```python
from build123d import *

# Parameters (mm, degrees)
RESSALTO_EXTRUS_O1_DEPTH = 102
ESBO_O3_R                = 1.5
CORTE_EXTRUS_O2_DEPTH    = 10


with BuildPart() as part:
    # Esboço1 → Ressalto-extrusão1 (new body)
    with BuildSketch(Plane.XY):
        Polygon((-21.132279289, 13.382352941), (-21.132279289, -6.617647059), (78.834377283, -9.19981162), align=None)
    extrude(amount=RESSALTO_EXTRUS_O1_DEPTH)

    # Esboço3 → Corte-extrusão2 (cut)
    with BuildSketch(Plane(origin=(-0.184911664, -7.158722975, 0), x_dir=(0.999666566, -0.025821646, 0), z_dir=(-0.025821646, -0.999666566, 0))):
        with Locations((4.045645474, 25)):
            Circle(ESBO_O3_R)
        with Locations((4.045645474, 77)):
            Circle(ESBO_O3_R)
    extrude(amount=-CORTE_EXTRUS_O2_DEPTH, mode=Mode.SUBTRACT)


solid = part.part
```
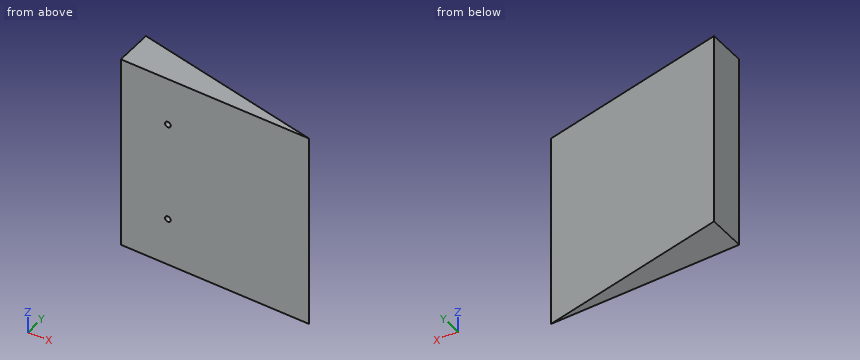
Input: part model. Units: mm. Frame: model coordinates. Coordinates: 2 decimals unless noted, no trailing zeros. Loops run counter-clockwise (first coordinate to the right, second up) from the corner with the lowest first, then second, coordinate; pieces in that order, holes last.
Q1. Section A-A, the plane y = 9.5. Return the cut outline in (x, z).
Results are:
outline: (-21.13, 0) - (-3.95, 0) - (-3.95, 102) - (-21.13, 102) - close
Q2. Section B-B, the plane z = 85.5. Return the cut outline in (x, y).
Results are:
outline: (-21.13, -6.62) - (78.83, -9.2) - (-21.13, 13.38) - close
Q3. Section D-D, the plane y = -1.5. Give the number of separate pieces and of enclosed holes in the cut face, and give its area (3 significant figures).
Results are:
separate pieces: 1
enclosed holes: 2
area: 6,710 mm2
Q4. Line query: line 1 along Z through (x, y) = (4.5, 2); line 2 along Y through (x, z) = (26, 71.5); line 3 along Y through (x, z) = (53.5, 32.5). Output: solid intervals per line, ascending.
Results are:
line 1: z = 0 to 23.55, 26.45 to 75.55, 78.45 to 102
line 2: y = -7.84 to 2.74
line 3: y = -8.55 to -3.48
Q5. Section C-C, the plane x = -7. Return the cut outline in (y, z), and give its area (3 significant figures).
Results are:
outline: (-6.98, 0) - (10.19, 0) - (10.19, 102) - (-6.98, 102) - close
area: 1,750 mm2
Q6. Contact query for flat-ended pins moving along their axis: pin 1 (12 mm diameter, centred on x = 36, y = -1, fed in from -Z); pin 2 (12 mm diameter, centred on x = 44.5, z = 84.5, fed in from +Y); pin 3 (5 mm diameter, centred on x = 59, z = 69.5, fed in from +Y); pin 4 (12 mm diameter, centred on x = -9, z = 51, fed in from -Y). Output: stop coordinate, or through.
Results are:
pin 1: stops at z = 0
pin 2: stops at y = -0.09
pin 3: stops at y = -4.15
pin 4: stops at y = -7.09
